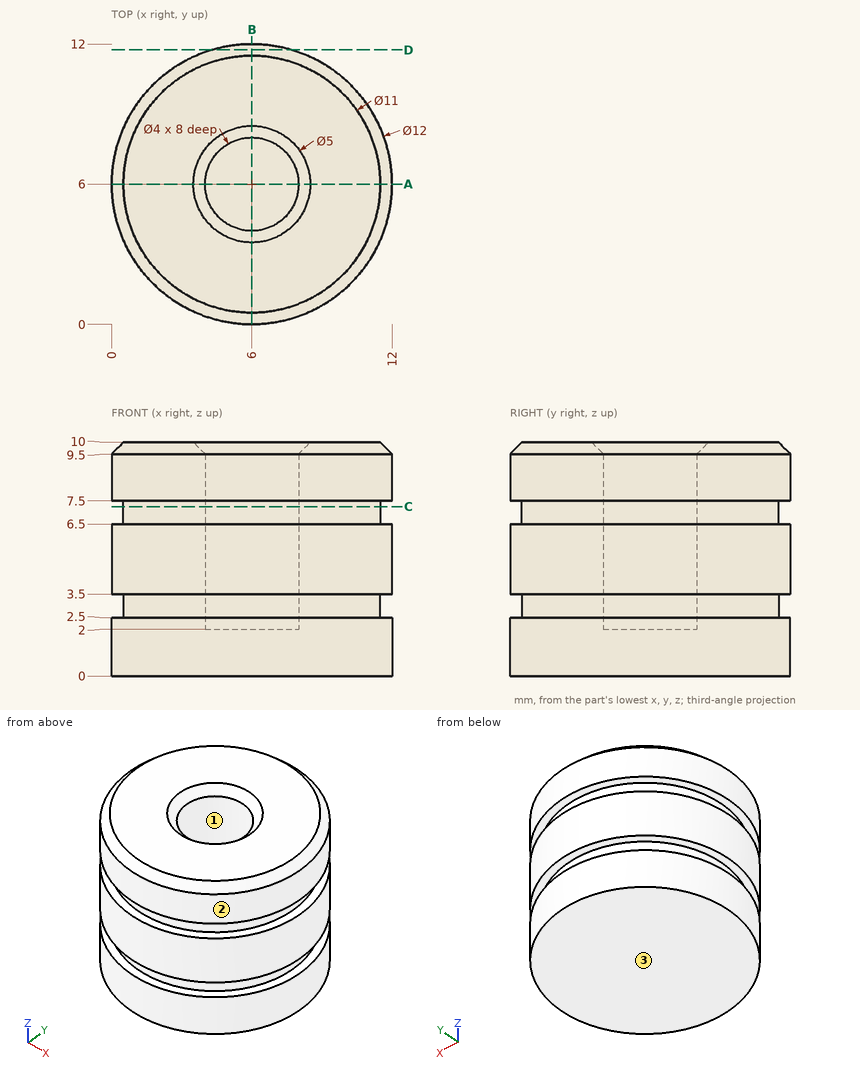
The figure shows three views and two pictorial views of one solid part (mm, origin at its lowest corner). Answer the questions. Coordinates: 2 decimals unless noted, no trailing zeros. Order: outer loops, then holes, each group sorted by start corner. A loop starts at its lowest first (then second) coordinate and runs counter-clockwise, first axis right, second up.
Q1. A cutting plane is placed at A-A, the plane y = 6. Write down the section's boundary in (x, z), and give its area (3 significant figures).
Q2. A cutting plane is placed at D-D, the plane y = 11.75. State how many separate pieces and enclosed holes the cut face has, and give its area (3 significant figures).
Q3. Given P1, Ø3, axis at x = 5.5, y = 5.5, coming from the +Z side; P2, Ø2, axis at x = 9.5, z = 5, coming from the +Y side; P3, Ø3.5, axis at x = 6, y = 6, coming from the +Z side, each flat-ended and moving along its own axis, determine where each tip first touches the part or whether it passes through.
Q4. For a pull along Y with two mould halves and no side action, classify the marked faces 1, 2 and 3 as pulls with the +Y half, pulls with the -Y half, needs draft (parallel to the pull), parting line crosses it, or undercut.
Q5. Consider line 1 (Y direction, x = 6, z = 4.75); line 2 (Z direction, x = 3.75, y = 11.25). Determine where each line is inside the solid, lowest interval first.
Q6. A cutting plane is placed at C-C, the plane z = 7.25. Write down the section's boundary in (x, y), and give its area (3 significant figures).
Answers follow:
1. outline: (0, 0) - (12, 0) - (12, 2.5) - (11.5, 2.5) - (11.5, 3.5) - (12, 3.5) - (12, 6.5) - (11.5, 6.5) - (11.5, 7.5) - (12, 7.5) - (12, 9.5) - (11.5, 10) - (8.5, 10) - (8, 9.5) - (8, 2) - (4, 2) - (4, 9.5) - (3.5, 10) - (0.5, 10) - (0, 9.5) - (0, 7.5) - (0.5, 7.5) - (0.5, 6.5) - (0, 6.5) - (0, 3.5) - (0.5, 3.5) - (0.5, 2.5) - (0, 2.5) - close
1. area: 85.5 mm2
2. separate pieces: 3
2. enclosed holes: 0
2. area: 26.3 mm2
3. P1: stops at z = 9.71
3. P2: stops at y = 11.45
3. P3: stops at z = 2
4. face 1: undercut
4. face 2: parting line crosses it
4. face 3: needs draft
5. line 1: y = 0 to 4, 8 to 12
5. line 2: z = 0 to 2.5, 3.5 to 6.5, 7.5 to 9.79
6. outline: circle Ø11 at (6, 6); hole circle Ø4 at (6, 6)
6. area: 82.5 mm2
